Build history of the part. All positions in model axes, mm. A direction names the side the tool comes from. Round coordinates to 2 decimals unless told otherwise and drop trailing zeros. Write each loop counter-clockwise with the first axis right and the second up, starting at its lowest first coordinate (ties: lowest second). Pieces come first, ordered by that corner, then holes.
1) Saw through at B-B (x = 28.5). State how many separate pieces and enclosed holes the cut face has, plus the area to 3 significant figures.
2) Pull direction X, two halves, no side cores. Call faces 1 (the flat face through (-34.189, -19.448, -2.719)), 2 (the flat face through (26.78, -14.33, -13)), 3 (the flat face through (-35, 17, -3)): +X half, -X half, draft (parallel to the pull), parting line (faces both ways), or undercut.
3) Wall check: probe 1 along Y at (x, z) = (28.5, -12.45); probe 2 along Y at (x, z) = (28.5, -0.5); probe 3 along Y at (x, z) = (-22.5, -12.4). Give the ranges that are in metal, low to high.
4) Flat gauge pins, fed straight in: pin 1 (7.5 mm diameter, centred on y = 10.5, z = -3, fed in from -X); pin 2 (1.7 mm diameter, centred on x = -21, y = 13.5, fed in from +Z); pin 3 (10 mm diameter, centred on x = 20.5, y = 3.5, fed in from -Z); pin 4 (18.5 mm diameter, centred on x = -17, y = -15, fed in from -Z). Where does each tip first touch, or does it go through?
5) Which spindle directions (+Z, -Z, +X, -X, +Y, -Y) get a long thin tool onto all of the face, cutting with end or side? Do faces 4 (the flat face through (26.064, 12.12, -5.061)), 5 (the flat face through (0, 0, 1.2)), 6 (the cylindrical face through (31.7, -15.9, -6.4)). Say none if no direction does.
6) Saw through at D-D (y = 18.5). Write the cut outline in (x, z), plus the area to 3 significant figures.
7) Saw through at C-C (x = 7.5). Write the cut outline in (y, z).
8) Saw through at A-A (z = -9.75). Write the cut outline in (x, y).
from build123d import *

# Parameters (mm, degrees)
SKETCH1_W           = 70
SKETCH1_H           = 45
BOSS_EXTRUDE1_DEPTH = 1.2
CUT_EXTRUDE1_DEPTH  = 11.2
SKETCH3_W           = 70
SKETCH3_H           = 45
SKETCH3_W_2         = 66.8
SKETCH3_H_2         = 41.8
BOSS_EXTRUDE2_DEPTH = 6.75
SKETCH4_R           = 4
BOSS_EXTRUDE3_DEPTH = 11.5
SKETCH5_R           = 4
SKETCH5_R_2         = 1.75
BOSS_EXTRUDE4_DEPTH = 1.5
SKETCH6_R           = 7
CUT_EXTRUDE2_DEPTH  = 11.5
CUT_EXTRUDE3_DEPTH  = 10
SKETCH8_R           = 4.75
CUT_EXTRUDE4_DEPTH  = 10


with BuildPart() as part:
    # Sketch1 → Boss-Extrude1 (new body)
    with BuildSketch(Plane.XY):
        Rectangle(SKETCH1_W, SKETCH1_H)
    extrude(amount=BOSS_EXTRUDE1_DEPTH)

    # Sketch2 → Cut-Extrude1 (cut)
    with BuildSketch(Plane.XY.offset(1.2)):
        Polygon((-20.883419246, 10.7), (-19.266838493, 13.5), (-20.883419246, 16.3), (-24.116580754, 16.3), (-25.733161507, 13.5), (-24.116580754, 10.7), align=None)
        Polygon((26.883419246, 10.7), (30.116580754, 10.7), (31.733161507, 13.5), (30.116580754, 16.3), (26.883419246, 16.3), (25.266838493, 13.5), align=None)
        Polygon((26.883419246, -16.3), (30.116580754, -16.3), (31.733161507, -13.5), (30.116580754, -10.7), (26.883419246, -10.7), (25.266838493, -13.5), align=None)
    extrude(amount=-CUT_EXTRUDE1_DEPTH, mode=Mode.SUBTRACT)

    # Sketch3 → Boss-Extrude2 (add)
    with BuildSketch(Plane(origin=(0, 0, 0), x_dir=(-1, 0, 0), z_dir=(0, 0, -1))):
        Rectangle(SKETCH3_W, SKETCH3_H)
        Rectangle(SKETCH3_W_2, SKETCH3_H_2, mode=Mode.SUBTRACT)
    extrude(amount=BOSS_EXTRUDE2_DEPTH)

    # Sketch4 → Boss-Extrude3 (add)
    with BuildSketch(Plane(origin=(0, 0, 0), x_dir=(-1, 0, 0), z_dir=(0, 0, -1))):
        with Locations((-28.5, 13.5)):
            Circle(SKETCH4_R)
        Polygon((-26.883419246, 10.7), (-30.116580754, 10.7), (-31.733161507, 13.5), (-30.116580754, 16.3), (-26.883419246, 16.3), (-25.266838493, 13.5), align=None, mode=Mode.SUBTRACT)
        with Locations((-28.5, -13.5)):
            Circle(SKETCH4_R)
        Polygon((-26.883419246, -10.7), (-25.266838493, -13.5), (-26.883419246, -16.3), (-30.116580754, -16.3), (-31.733161507, -13.5), (-30.116580754, -10.7), align=None, mode=Mode.SUBTRACT)
        with Locations((22.5, 13.5)):
            Circle(SKETCH4_R)
        Polygon((24.116580754, 10.7), (20.883419246, 10.7), (19.266838493, 13.5), (20.883419246, 16.3), (24.116580754, 16.3), (25.733161507, 13.5), align=None, mode=Mode.SUBTRACT)
    extrude(amount=BOSS_EXTRUDE3_DEPTH)

    # Sketch5 → Boss-Extrude4 (add)
    with BuildSketch(Plane(origin=(0, 0, -11.5), x_dir=(-1, 0, 0), z_dir=(0, 0, -1))):
        with Locations((-28.5, -13.5)):
            Circle(SKETCH5_R)
        with Locations((-28.5, -13.5)):
            Circle(SKETCH5_R_2, mode=Mode.SUBTRACT)
        with Locations((22.5, 13.5)):
            Circle(SKETCH5_R)
        with Locations((22.5, 13.5)):
            Circle(SKETCH5_R_2, mode=Mode.SUBTRACT)
        with Locations((-28.5, 13.5)):
            Circle(SKETCH5_R)
        with Locations((-28.5, 13.5)):
            Circle(SKETCH5_R_2, mode=Mode.SUBTRACT)
    extrude(amount=BOSS_EXTRUDE4_DEPTH)

    # Sketch6 → Cut-Extrude2 (cut)
    with BuildSketch(Plane(origin=(35, 0, 0), x_dir=(0, 0, -1), z_dir=(1, 0, 0))):
        with Locations((6.75, 1.13)):
            Circle(SKETCH6_R)
    extrude(amount=-CUT_EXTRUDE2_DEPTH, mode=Mode.SUBTRACT)

    # Sketch7 → Cut-Extrude3 (cut)
    with BuildSketch(Plane.XY.offset(1.2)):
        Polygon((-35, 11.02), (-33.4, 11.943760431), (-33.4, -19.903760431), (-35, -18.98), align=None)
    extrude(amount=-CUT_EXTRUDE3_DEPTH, mode=Mode.SUBTRACT)

    # Sketch8 → Cut-Extrude4 (cut)
    with BuildSketch(Plane.XY.offset(1.2)):
        with Locations((7.5, 0.5)):
            Circle(SKETCH8_R)
    extrude(amount=-CUT_EXTRUDE4_DEPTH, mode=Mode.SUBTRACT)


solid = part.part
Evaluation:
1. separate pieces: 3
1. enclosed holes: 0
1. area: 130 mm2
2. face 1: undercut
2. face 2: draft
2. face 3: -X half
3. probe 1: y = -17.5 to -15.25, -11.75 to -9.5, 9.5 to 11.75, 15.25 to 17.5
3. probe 2: y = -22.5 to -20.9, -17.5 to -16.3, -10.7 to -9.5, 9.5 to 10.7, 16.3 to 17.5, 20.9 to 22.5
3. probe 3: y = 9.5 to 11.75, 15.25 to 17.5
4. pin 1: stops at x = -35
4. pin 2: stops at z = -11.5
4. pin 3: stops at z = 0
4. pin 4: stops at z = -6.75
5. face 4: +Z
5. face 5: +Z, +X, -X, +Y, -Y
5. face 6: -Z
6. outline: (-35, -6.75) - (-33.4, -6.75) - (-33.4, 0) - (33.4, 0) - (33.4, -6.75) - (35, -6.75) - (35, 1.2) - (-35, 1.2) - close
6. area: 106 mm2
7. outline: (-22.5, -6.75) - (-20.9, -6.75) - (-20.9, 0) - (-4.25, 0) - (-4.25, 1.2) - (-22.5, 1.2) - close; (5.25, 0) - (20.9, 0) - (20.9, -6.75) - (22.5, -6.75) - (22.5, 1.2) - (5.25, 1.2) - close
8. outline: circle Ø8 at (-22.5, 13.5); circle Ø8 at (28.5, -13.5); circle Ø8 at (28.5, 13.5); hole (-25.73, 13.5) - (-24.12, 10.7) - (-20.88, 10.7) - (-19.27, 13.5) - (-20.88, 16.3) - (-24.12, 16.3) - close; hole (25.27, -13.5) - (26.88, -16.3) - (30.12, -16.3) - (31.73, -13.5) - (30.12, -10.7) - (26.88, -10.7) - close; hole (25.27, 13.5) - (26.88, 10.7) - (30.12, 10.7) - (31.73, 13.5) - (30.12, 16.3) - (26.88, 16.3) - close
